Build history of the part. All positions in model axes, mm. A direction names the side the tool comes from. Coordinates: 2 decimals unless noted, no trailing zeros. Order: outer loops, then holes, each group sorted by start corner. A loop starts at its lowest first (then second) coordinate and runs counter-clockwise, first axis right, second up. Notation, with made-up numbers: (-5, -16) - (0, -16) arc R8 cw to (0, -10) - close; hole circle Ø9 at (30.25, -29). An arc over 180 degrees is marked (long way). One line per item, written item: value.
from build123d import *

# Parameters (mm, degrees)
BOSS_EXTRUDE1_DEPTH        = 6
BOSS_EXTRUDE2_DEPTH        = 6
BOSS_EXTRUDE3_START        = 18
SKETCH3_R                  = 30
BOSS_EXTRUDE3_DEPTH        = 18
F_10_0_10_DIAMETER_HOLE1_D = 10
M45_CLEARANCE_HOLE1_D      = 50


with BuildPart() as part:
    # Sketch1 → Boss-Extrude1 (new body)
    with BuildSketch(Plane(origin=(0, 12, 0), x_dir=(1, 0, 0), z_dir=(0, 1, 0))):
        with BuildLine():
            Line((-45.687618347, -8), (-28.91366459, -8))
            ThreePointArc((-28.91366459, -8), (-28.275380984, -10.025109984), (-27.49545417, -12))
            Line((-27.49545417, -12), (-9.16515139, -54))
            ThreePointArc((-9.16515139, -54), (0, -60), (9.16515139, -54))
            Line((9.16515139, -54), (27.49545417, -12))
            ThreePointArc((27.49545417, -12), (28.275380984, -10.025109984), (28.91366459, -8))
            Line((28.91366459, -8), (45.687618347, -8))
            ThreePointArc((45.687618347, -8), (50.272203932, 0), (45.687618347, 8))
            Line((45.687618347, 8), (28.91366459, 8))
            ThreePointArc((28.91366459, 8), (0, 30), (-28.91366459, 8))
            Line((-28.91366459, 8), (-45.687618347, 8))
            ThreePointArc((-45.687618347, 8), (-50.272203932, 0), (-45.687618347, -8))
        make_face()
    extrude(amount=-BOSS_EXTRUDE1_DEPTH)

    # Sketch2 → Boss-Extrude2 (add)
    with BuildSketch(Plane.XZ.offset(-6)):
        with BuildLine():
            Line((-15.16668005, -25.883813789), (-45.687618347, -8))
            ThreePointArc((-45.687618347, -8), (-50.272203932, 0), (-45.687618347, 8))
            Line((-45.687618347, 8), (-23.590216691, 20.948023176))
            Line((-23.590216691, 20.948023176), (-9.16515139, 54))
            ThreePointArc((-9.16515139, 54), (0, 60), (9.16515139, 54))
            Line((9.16515139, 54), (23.590216691, 20.948023176))
            Line((23.590216691, 20.948023176), (45.687618347, 8))
            ThreePointArc((45.687618347, 8), (50.272203932, 0), (45.687618347, -8))
            Line((45.687618347, -8), (15.16668005, -25.883813789))
            ThreePointArc((15.16668005, -25.883813789), (0, -30), (-15.16668005, -25.883813789))
        make_face()
    extrude(amount=BOSS_EXTRUDE2_DEPTH)

    # Sketch3 → Boss-Extrude3 (add)
    with BuildSketch(Plane(origin=(0, 12, 0), x_dir=(-1, 0, 0), z_dir=(0, 1, 0)).offset(BOSS_EXTRUDE3_START)):
        with Locations(Location((0, 0, 0), (0, 0, 90))):
            Circle(SKETCH3_R)
    extrude(amount=-BOSS_EXTRUDE3_DEPTH)

    # Ø10.0 (10) Diameter Hole1 (through all)
    with Locations(Plane(origin=(0, 12, 0), x_dir=(1, 0, 0), z_dir=(0, 1, 0))):
        with Locations((-41, 0), (41, 0), (0, -50)):
            Hole(F_10_0_10_DIAMETER_HOLE1_D / 2)

    # M45 Clearance Hole1 (through all)
    with Locations(Plane(origin=(0, 30, 0), x_dir=(1, 0, 0), z_dir=(0, 1, 0))):
        with Locations((0, 0)):
            Hole(M45_CLEARANCE_HOLE1_D / 2)


solid = part.part
1. Two-plate mould, pull along X, no slides. Class faces 1 (the face through (0.2, 0, 25.2)), 2 (the face through (-36, 6, 0)), 3 (the face through (30.641, 3.042, -16.817)), 4 (the face through (-50.27, 6.08, -0.14)): pulls with the +X half, pulls with the -X half, needs draft (parallel to the pull), parting line crosses it, or undercut.
Values found:
face 1: needs draft
face 2: undercut
face 3: pulls with the +X half
face 4: pulls with the -X half
2. Flat gauge pins, fed straight in: P1, Ø8, axis at x = 41, z = 0, coming from the -Y side; P2, Ø6.5, axis at x = -39.5, z = 12.5, coming from the +Y side; P3, Ø6.5, axis at x = -41, y = 10, coming from the +Z side; P4, Ø8, axis at x = 43.5, z = -0.5, coming from the +Y side. Where does each tip first touch, or does it go through?
Values found:
P1: passes through
P2: stops at y = 6
P3: stops at z = 8
P4: stops at y = 12
3. Probe line 1 along Z through (x, y) = (0, 9); line 2 along Z through (x, y) = (0, 21); line 3 along Y through (x, z) = (-9, 39.5). List the from-to ranges inside material, lowest first.
Values found:
line 1: z = -30 to -25, 25 to 45, 55 to 60
line 2: z = -30 to -25, 25 to 30
line 3: y = 0 to 12
4. Band-saw the part on A-A, the plane z = 0. Give the cut face in (x, y).
Values found:
outline: (-50.27, 0) - (-46, 0) - (-46, 12) - (-50.27, 12) - close; (-36, 0) - (-25, 0) - (-25, 30) - (-30, 30) - (-30, 12) - (-36, 12) - close; (25, 0) - (36, 0) - (36, 12) - (30, 12) - (30, 30) - (25, 30) - close; (46, 0) - (50.27, 0) - (50.27, 12) - (46, 12) - close
5. Band-saw the part on D-D, the plane z = -10. Give the cut face in (x, y), and give its area (3 significant figures).
Values found:
outline: (-42.27, 0) - (-22.91, 0) - (-22.91, 30) - (-28.28, 30) - (-28.28, 6) - (-42.27, 6) - close; (22.91, 0) - (42.27, 0) - (42.27, 6) - (28.28, 6) - (28.28, 30) - (22.91, 30) - close
area: 490 mm2
6. Band-saw the part on C-C, the plane y = 2.75. Give the cut face in (x, z).
Values found:
outline: (-45.69, -8) - (-15.17, -25.88) arc R30 ccw to (15.17, -25.88) - (45.69, -8) arc R9.27 ccw to (45.69, 8) - (23.59, 20.95) - (9.17, 54) arc R10 ccw to (-9.17, 54) - (-23.59, 20.95) - (-45.69, 8) arc R9.27 ccw to start; hole circle Ø10 at (-41, 0); hole circle Ø50 at (0, 0); hole circle Ø10 at (0, 50); hole circle Ø10 at (41, 0)
7. Band-saw the part on B-B, the plane x = 0. Give the cut face in (y, z), and give its area (3 significant figures).
Values found:
outline: (0, -30) - (30, -30) - (30, -25) - (0, -25) - close; (0, 25) - (30, 25) - (30, 30) - (12, 30) - (12, 45) - (0, 45) - close; (0, 55) - (12, 55) - (12, 60) - (0, 60) - close
area: 540 mm2
8. 3-axis set-ups, long thin cutter, end or side, ignore diameter. For faces 5 (the face through (-31, 6, -14)), 6 (the face through (37, 9, 8)), 7 (the face through (37, 9, -8)), 8 (the face through (-37, 9, 8)): which of +Z, -Z, +X, -X, +Y, -Y reach the whole face in a straight line?
Values found:
face 5: -Z, -X, +Y
face 6: +Z, +X, +Y
face 7: -Z, +X, +Y
face 8: +Z, -X, +Y
